Read the model definition and answer for the solid it produces. Units are mm, in the model's axes. Face numbers are marked on the shaded views. A direction names the side the tool comes from. Give positions to 0.01 mm unless a question says otherwise; leave off trailing zeros. Use a Markdown table: item, result. Add a question column.
Item 1: Given P1, Ø4, axis at x = 23, z = 7, coming from the +Y side; P2, Ø1, axis at x = 5, z = 2.5, coming from the -Y side; P3, Ø1.5, axis at y = -2, z = 3, coming from the -X side, each flat-ended and moving along its own axis, determine where each tip first touches the part or whether it passes through.
Item 2: A cutting plane is placed at A-A on z = 2.25. Count the separate pieces of the cut face and the enclosed holes in it, then the cut area to 3 significant figures.
Item 3: For the marked faces 3 and 4, determine the directions among +Z, -Z, +X, -X, +Y, -Y from which every point of the face is accessible in a straight line to the end or side of a thin tool.
Item 4: Consider probe 1 along Y at (x, z) = (33, 2); probe 2 along Y at (x, z) = (26, 0.75); probe 3 along Z at (x, y) = (-21, -6). Determine where each line is inside the solid, lowest interval first. Write a range as [from, to].
Item 5: The mould has two halves that part along X. Classify the marked faces 1 and 2: pulls with the +X half, pulls with the -X half, needs draft (parallel to the pull), parting line crosses it, or undercut.
Autodesk Fusion 360 part; units mm, degrees
sketch "Sketch1" plane through (0, 0, 0) normal (0, 0, 1) x (1, 0, 0)
  circle A0 centre (0, 0) radius 45
  circle A1 centre (0, 0) radius 40
  dimension "d1" = 90
  dimension "d2" = -5
extrude "Extrude1" add sketch "Sketch1" along normal blind 8
extrude "Extrude2" add sketch "Sketch1" along normal blind 5 contours A1
sketch "Sketch2" plane through (0, 0, 5) normal (0, 0, 1) x (-1, 0, 0)
  line L0 (9.7065, -15.2032) -> (10.5595, -24.1789)
  line L1 (10.5595, -24.1789) -> (19.3595, -26.1413)
  line L2 (19.3595, -26.1413) -> (23.9453, -18.3784)
  line L3 (23.9453, -18.3784) -> (17.9794, -11.6183)
  line L4 (17.9794, -11.6183) -> (9.7065, -15.2032)
  line L5 (2.3064, 1.7998) -> (3.1593, -7.176)
  line L6 (16.5451, -1.3755) -> (10.5792, 5.3847)
  line L7 (10.5792, 5.3847) -> (2.3064, 1.7998)
  line L8 (3.1593, -7.176) -> (11.9594, -9.1384)
  line L9 (11.9594, -9.1384) -> (16.5451, -1.3755)
  line L10 (-0.1005, -5.1751) -> (-9.1149, -5.3544)
  line L11 (-11.73, -13.983) -> (-4.3318, -19.1365)
  line L12 (-4.3318, -19.1365) -> (2.8556, -13.6929)
  line L13 (-9.1149, -5.3544) -> (-11.73, -13.983)
  line L14 (2.8556, -13.6929) -> (-0.1005, -5.1751)
  line L15 (17.5268, 24.1869) -> (14.993, 15.534)
  line L16 (22.4394, 10.4504) -> (29.5752, 15.9614)
  line L17 (29.5752, 15.9614) -> (26.5391, 24.451)
  line L18 (14.993, 15.534) -> (22.4394, 10.4504)
  line L19 (26.5391, 24.451) -> (17.5268, 24.1869)
  line L20 (33.7221, -3.6823) -> (30.2498, 4.6384)
  line L21 (30.2498, 4.6384) -> (21.2633, 3.9073)
  line L22 (19.1816, -4.8653) -> (26.8816, -9.5559)
  line L23 (21.2633, 3.9073) -> (19.1816, -4.8653)
  line L24 (26.8816, -9.5559) -> (33.7221, -3.6823)
  line L25 (7.0524, -33.7264) -> (7.1423, -24.7107)
  line L26 (7.1423, -24.7107) -> (-1.4044, -21.8392)
  line L27 (-1.5498, -36.427) -> (7.0524, -33.7264)
  line L28 (-1.4044, -21.8392) -> (-6.7764, -29.0802)
  line L29 (-6.7764, -29.0802) -> (-1.5498, -36.427)
  line L30 (8.7825, 20.5049) -> (-0.2283, 20.1944)
  line L31 (4.7548, 6.4834) -> (11.8623, 12.031)
  line L32 (11.8623, 12.031) -> (8.7825, 20.5049)
  line L33 (-0.2283, 20.1944) -> (-2.7176, 11.5287)
  line L34 (-2.7176, 11.5287) -> (4.7548, 6.4834)
  line L35 (-9.6613, 12.6209) -> (-18.1524, 9.5888)
  line L36 (-4.1538, 5.4824) -> (-9.6613, 12.6209)
  line L37 (-17.8926, 0.5764) -> (-9.241, -1.9616)
  line L38 (-9.241, -1.9616) -> (-4.1538, 5.4824)
  line L39 (-18.1524, 9.5888) -> (-17.8926, 0.5764)
  line L40 (-29.0638, -18.1025) -> (-20.4014, -15.6016)
  line L41 (-20.1031, -6.5904) -> (-28.5811, -3.522)
  line L42 (-28.5811, -3.522) -> (-34.1191, -10.6369)
  line L43 (-34.1191, -10.6369) -> (-29.0638, -18.1025)
  line L44 (-20.4014, -15.6016) -> (-20.1031, -6.5904)
  line L45 (-20.2979, 29.9068) -> (-22.3795, 21.1342)
  line L46 (-14.6796, 16.4435) -> (-7.8391, 22.3171)
  line L47 (-22.3795, 21.1342) -> (-14.6796, 16.4435)
  line L48 (-7.8391, 22.3171) -> (-11.3114, 30.6379)
  line L49 (-11.3114, 30.6379) -> (-20.2979, 29.9068)
  line L50 (-22.4664, 11.7936) -> (-31.0997, 14.393)
  line L51 (-31.0997, 14.393) -> (-36.2397, 6.9854)
  line L52 (-30.783, -0.1921) -> (-22.2706, 2.7796)
  line L53 (-22.2706, 2.7796) -> (-22.4664, 11.7936)
  line L54 (-36.2397, 6.9854) -> (-30.783, -0.1921)
  line L55 (-4.3507, 26.0684) -> (3.3493, 21.3777)
  line L56 (10.1898, 27.2513) -> (6.7174, 35.5721)
  line L57 (3.3493, 21.3777) -> (10.1898, 27.2513)
  line L58 (-2.2691, 34.841) -> (-4.3507, 26.0684)
  line L59 (6.7174, 35.5721) -> (-2.2691, 34.841)
  line L60 (-15.175, -31.8449) -> (-8.3345, -25.9713)
  line L61 (-11.8069, -17.6506) -> (-20.7934, -18.3817)
  line L62 (-22.875, -27.1543) -> (-15.175, -31.8449)
  line L63 (-8.3345, -25.9713) -> (-11.8069, -17.6506)
  line L64 (-20.7934, -18.3817) -> (-22.875, -27.1543)
  point P0 (16.31, -19.104)
  point P1 (8.9099, -2.1011)
  point P2 (-4.4843, -11.4684)
  point P3 (22.2147, 18.1167)
  point P4 (26.2597, -1.9116)
  point P5 (0.8928, -29.1567)
  point P6 (4.4907, 14.1485)
  point P7 (-11.8202, 5.2614)
  point P8 (-26.4537, -10.8907)
  point P9 (-15.3015, 24.0879)
  point P10 (-28.5719, 7.1519)
  point P11 (6.7127, 26.555)
  point P12 (2.7273, 29.0221)
  point P13 (-15.797, -24.2006)
extrude "Extrude3" cut sketch "Sketch2" against normal through all
fillet "Fillet1" radius 3.793 1 edges at (-41.9547, -16.2727, 8)
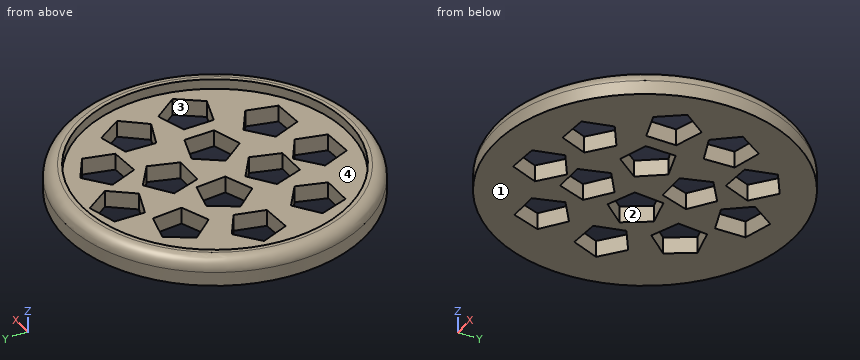
Filled in:
| question | item | result |
|---|---|---|
| 1 | P1 | y = 39.19 |
| 1 | P2 | y = -44.77 |
| 1 | P3 | x = -44.98 |
| 2 | separate pieces | 1 |
| 2 | enclosed holes | 13 |
| 2 | area | 4,540 mm² |
| 3 | face 3 | +Z, -Z |
| 3 | face 4 | +Z |
| 4 | probe 1 | [-30.59, -11.65], [-2.72, 9.2], [12.29, 30.59] |
| 4 | probe 2 | [-36.73, -12.86], [-1.48, 4.46], [17.22, 36.73] |
| 4 | probe 3 | [0, 5] |
| 5 | face 1 | needs draft |
| 5 | face 2 | undercut |
